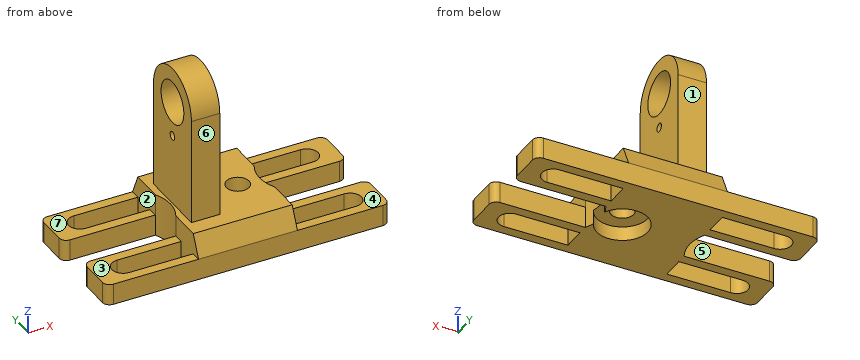
```python
from build123d import *

# Parameters (mm, degrees)
EXTRUDE_1_DEPTH     = 3
EXTRUDE_START       = -3
EXTRUDE_2_DEPTH     = 6
EXTRUDE_START_2     = -2
SKETCH_3_R          = 3
SKETCH_3_R_2        = 0.6
EXTRUDE_3_DEPTH     = 4
FILLET_2_R          = 1
EXTRUDE_4_DEPTH     = 13.942167231
SKETCH_8_R          = 1.6
CUT_EXTRUDE_1_DEPTH = 30.596473185
SKETCH_9_R          = 3.6
CUT_EXTRUDE_2_DEPTH = 2


with BuildPart() as part:
    # 草图1 → 凸台-拉伸1 (new body)
    with BuildSketch(Plane.XY):
        with BuildLine():
            Line((20, 8.715), (20, 2.715))
            Line((20, 2.715), (6.971083616, 2.715))
            ThreePointArc((6.971083616, 2.715), (6.285, 0), (6.971083616, -2.715))
            Line((6.971083616, -2.715), (20, -2.715))
            Line((20, -2.715), (20, -8.715))
            Line((20, -8.715), (-20, -8.715))
            Line((-20, -8.715), (-20, -2.715))
            Line((-20, -2.715), (-6.971083616, -2.715))
            ThreePointArc((-6.971083616, -2.715), (-6.285, 0), (-6.971083616, 2.715))
            Line((-6.971083616, 2.715), (-20, 2.715))
            Line((-20, 2.715), (-20, 8.715))
            Line((-20, 8.715), (20, 8.715))
        make_face()
        with BuildLine():
            Line((16, 4.115), (-16, 4.115))
            ThreePointArc((-16, 4.115), (-17.6, 5.715), (-16, 7.315))
            Line((-16, 7.315), (16, 7.315))
            ThreePointArc((16, 7.315), (17.6, 5.715), (16, 4.115))
        make_face(mode=Mode.SUBTRACT)
        with BuildLine():
            Line((16, -7.315), (-16, -7.315))
            ThreePointArc((-16, -7.315), (-17.6, -5.715), (-16, -4.115))
            Line((-16, -4.115), (16, -4.115))
            ThreePointArc((16, -4.115), (17.6, -5.715), (16, -7.315))
        make_face(mode=Mode.SUBTRACT)
    extrude(amount=EXTRUDE_1_DEPTH)

    # 草图2 → 凸台-拉伸2 (add)
    with BuildSketch(Plane.XY.offset(3).offset(EXTRUDE_START)):
        with BuildLine():
            Line((-6.971083616, 2.715), (-6.971083616, 4.115))
            Line((-6.971083616, 4.115), (-6.971083616, 7.315))
            Line((-6.971083616, 7.315), (6.971083616, 7.315))
            Line((6.971083616, 7.315), (6.971083616, 4.115))
            Line((6.971083616, 4.115), (6.971083616, 2.715))
            ThreePointArc((6.971083616, 2.715), (6.285, 0), (6.971083616, -2.715))
            Line((6.971083616, -2.715), (6.971083616, -4.115))
            Line((6.971083616, -4.115), (6.971083616, -7.315))
            Line((6.971083616, -7.315), (-6.971083616, -7.315))
            Line((-6.971083616, -7.315), (-6.971083616, -4.115))
            Line((-6.971083616, -4.115), (-6.971083616, -2.715))
            ThreePointArc((-6.971083616, -2.715), (-6.285, 0), (-6.971083616, 2.715))
        make_face()
    extrude(amount=EXTRUDE_2_DEPTH)

    # 草图3 → 凸台-拉伸3 (add)
    with BuildSketch(Plane(origin=(0, 0, 0), x_dir=(0, 0, -1), z_dir=(1, 0, 0)).offset(EXTRUDE_START_2)):
        with BuildLine():
            Line((-6, 5), (-21, 5))
            ThreePointArc((-21, 5), (-26, 0), (-21, -5))
            Line((-21, -5), (-6, -5))
            Line((-6, -5), (-6, 5))
        make_face()
        with Locations((-21, 0)):
            Circle(SKETCH_3_R, mode=Mode.SUBTRACT)
        with Locations((-16, 0)):
            Circle(SKETCH_3_R_2, mode=Mode.SUBTRACT)
    extrude(amount=-EXTRUDE_3_DEPTH)

    # 圆角2
    fillet_2_edges = [part.edges().sort_by_distance(p)[0] for p in [
        (-20, -8.715, 1.5),
        (-20, -2.715, 1.5),
        (-20, 2.715, 1.5),
        (-20, 8.715, 1.5),
        (20, 8.715, 1.5),
        (20, 2.715, 1.5),
        (20, -2.715, 1.5),
        (20, -8.715, 1.5),
    ]]
    fillet(fillet_2_edges, radius=FILLET_2_R)

    # 草图6 → 凸台-拉伸4 (add)
    with BuildSketch(Plane(origin=(6.971083616, 0, 0), x_dir=(0, 0, -1), z_dir=(1, 0, 0))):
        Polygon((-6, 7.315), (-3, 8.715), (-3, 7.315), align=None)
        Polygon((-3, -7.315), (-6, -7.315), (-3, -8.715), align=None)
    extrude(amount=-EXTRUDE_4_DEPTH)

    # 草图8 → 切除-拉伸1 (cut, through all)
    with BuildSketch(Plane.XY.offset(6)):
        with Locations((3.2, 0)):
            Circle(SKETCH_8_R)
    extrude(amount=-CUT_EXTRUDE_1_DEPTH, mode=Mode.SUBTRACT)

    # 草图9 → 切除-拉伸2 (cut)
    with BuildSketch(Plane(origin=(0, 0, 0), x_dir=(-1, 0, 0), z_dir=(0, 0, -1))):
        with Locations((-3.2, 0)):
            Circle(SKETCH_9_R)
    extrude(amount=-CUT_EXTRUDE_2_DEPTH, mode=Mode.SUBTRACT)


solid = part.part
```
Read the model definition and answer for the solid it produces. Units are mm, in the model's axes. Face numbers are marked on the shaded views. A direction names the side the tool comes from. Coordinates: 2 decimals unless noted, no trailing zeros. Loops run counter-clockwise (first coordinate to the right, second up) from the corner with the lowest first, then second, coordinate; pieces in that order, holes last. Notation, with made-up numbers: (23, -11.75) -> (33, -11.75) arc R18 cw to (33, 0.25) -> close; hole circle Ø7 at (87.5, 37). An arc over 180 degrees is marked (long way). Return JSON: item names as keys, results as strings.
Item 1: Find section B-B (x = -8). Determine the outline of the cut face in (y, z) (3 decimals), plus the area to 3 significant figures.
Answers:
{"outline": "(-8.715, 0) -> (-7.315, 0) -> (-7.315, 3) -> (-8.715, 3) -> close; (-4.115, 0) -> (-2.715, 0) -> (-2.715, 3) -> (-4.115, 3) -> close; (2.715, 0) -> (4.115, 0) -> (4.115, 3) -> (2.715, 3) -> close; (7.315, 0) -> (8.715, 0) -> (8.715, 3) -> (7.315, 3) -> close", "area": "16.8 mm2"}
Item 2: Find section C-C (z = 16). Determine the outline of the cut face in (x, y).
Answers:
{"outline": "(-6, -5) -> (-2, -5) -> (-2, -0.6) -> (-6, -0.6) -> close; (-6, 0.6) -> (-2, 0.6) -> (-2, 5) -> (-6, 5) -> close"}
Item 3: Flat-ended cylindrical pins translate along their axes: P1, Ø4.5, axis at x = -3.5, z = 11, coming from the -Y side; P2, Ø3, axis at x = 14.5, y = -7, coming from the +Z side; P3, Ø3, axis at y = -3.5, z = 8.5, coming from the +X side; P4, Ø3, axis at x = 16, y = -7, coming from the -Z side. Find the tip coordinate at first contact, or state that the pin passes through.
Answers:
{"P1": "stops at y = -5", "P2": "stops at z = 3", "P3": "stops at x = -2", "P4": "stops at z = 0"}
Item 4: For the marked faces 4, 5, 6 and 7, determine the directions among +Z, -Z, +X, -X, +Y, -Y from which every point of the face is accessible in a straight line to the end or side of a thin tool.
Answers:
{"face 4": "+Z, +X, +Y, -Y", "face 5": "+Z, -Z, -X", "face 6": "+Z, +X, -X, -Y", "face 7": "+Z, -X, +Y, -Y"}
Item 5: Find section A-A (x = 3.2). Determine the outline of the cut face in (y, z) (3 decimals), plus the area to 3 significant figures.
Answers:
{"outline": "(-8.715, 0) -> (-3.6, 0) -> (-3.6, 2) -> (-1.6, 2) -> (-1.6, 6) -> (-7.315, 6) -> (-8.715, 3) -> close; (1.6, 2) -> (3.6, 2) -> (3.6, 0) -> (8.715, 0) -> (8.715, 3) -> (7.315, 6) -> (1.6, 6) -> close", "area": "73.2 mm2"}
Item 6: For a pull along Y with two mould halves and no side action, classify the marked faces 1, 2 and 3 as +Y half, -Y half, draft (parallel to the pull), parting line (faces both ways), or undercut.
Answers:
{"face 1": "+Y half", "face 2": "undercut", "face 3": "draft"}
Item 7: Find section D-D (y = 0). Determine the outline of the cut face in (x, z) (3 decimals).
Answers:
{"outline": "(-6.285, 0) -> (-0.4, 0) -> (-0.4, 2) -> (1.6, 2) -> (1.6, 6) -> (-2, 6) -> (-2, 15.4) -> (-6, 15.4) -> (-6, 6) -> (-6.285, 6) -> close; (-6, 16.6) -> (-2, 16.6) -> (-2, 18) -> (-6, 18) -> close; (-6, 24) -> (-2, 24) -> (-2, 26) -> (-6, 26) -> close; (4.8, 2) -> (6.285, 2) -> (6.285, 6) -> (4.8, 6) -> close"}
Item 8: Find the intervals of material crossed by probe 1 along Y at (x, z) = (-3, 16); probe 2 along Y at (x, z) = (-4.25, 21); probe 3 along X at (y, z) = (-6, 2.75), in increasing order.
Answers:
{"probe 1": "y = -5 to -0.6, 0.6 to 5", "probe 2": "y = -5 to -3, 3 to 5", "probe 3": "x = -20 to -17.57, -6.97 to 6.97, 17.57 to 20"}
